Source: CAD feature listing. Evaluate the final solid. Frame: model axes, mm. Face numbers are marked on the shaded views. A direction names the side the tool comes from. Round coordinates to 2 decimals unless told otherwise and drop trailing zeros. Order: outer loops, then holes, each group sorted by start corner. A loop starts at its lowest first (then second) coordinate and runs counter-clockwise, first axis right, second up. Notation, with made-up numbers: M -19.75,-18.75 L 10.25,-18.75 A20 ccw 10.25,11.25 Z; hole C 47,15 d1. An arc over 180 degrees is marked long. Answer in a Markdown table with one row per item. Add a question column.
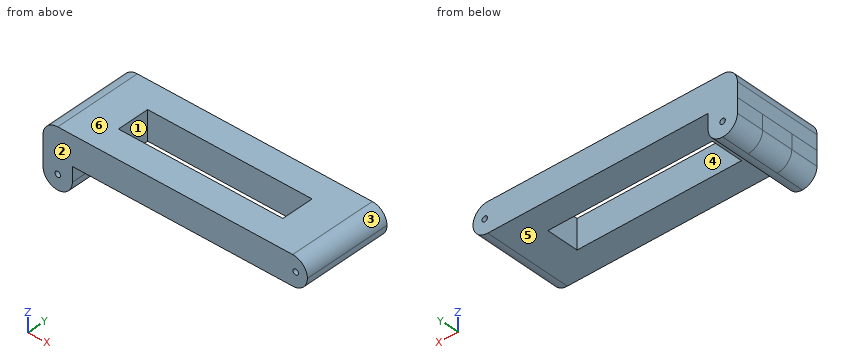
Autodesk Fusion 360 part; units mm, degrees
sketch "Esquisse1" plane through (0, 0, 0) normal (0, 0, 1) x (1, 0, 0)
  line L0 (-58.016, 25) -> (31.984, 25)
  line L1 (31.984, 25) -> (31.984, -5)
  line L2 (31.984, -5) -> (-58.016, -5)
  line L3 (-58.016, -5) -> (-58.016, 25)
  dimension "d1" = 90
  dimension "d2" = 30
extrude "Extrusion1" add sketch "Esquisse1" along normal blind 10
sketch "Esquisse11" plane through (0, 0, 0) normal (0, 1, 0) x (1, 0, 0)
  line L0 (-58.0163, -0.0111) -> (-48.0163, -0.0111)
  line L1 (-48.0163, -0.0111) -> (-48.0163, 9.9889)
  line L2 (-48.0163, 9.9889) -> (-58.0163, 9.9889)
  line L3 (-58.0163, 9.9889) -> (-58.0163, -0.0111)
  dimension "d56" = 10
  dimension "d57" = 10
extrude "Extrusion7" add sketch "Esquisse11" along normal blind 25 and the other way blind 5
sketch "Esquisse5" plane through (0, -5, 0) normal (0, -1, 0) x (1, 0, 0)
  line L0 (-48.0163, 0) -> (31.984, 0)
  line L1 (31.984, 0) -> (31.984, 10)
  line L2 (31.984, 10) -> (-58.016, 10)
  line L3 (-58.016, 10) -> (-58.016, 0.0111)
  circle A0 centre (28, 5) radius 6.5
  circle A1 centre (-53.0143, -5.2112) radius 7.25
  line L4 (-58.0163, 0.0111) -> (-58.0163, -9.9889)
  line L5 (-58.0163, -9.9889) -> (-48.0163, -9.9889)
  line L6 (-48.0163, -9.9889) -> (-48.0163, 0)
  line L7 (-58.016, 0.0111) -> (-58.0163, 0.0111)
  dimension "d11" = 13
  dimension "d46" = 14.5
sketch "Esquisse7" plane through (0, 0, 10) normal (0, 0, 1) x (-1, 0, 0)
  line L0 (-31.984, 5) -> (-31.984, -25)
  line L1 (-31.984, -25) -> (58.016, -25)
  line L2 (58.016, 5) -> (-31.984, 5)
  line L3 (41.016, -15.609) -> (-14.984, -15.609)
  line L4 (-14.984, -15.609) -> (-14.984, -4.609)
  line L5 (-14.984, -4.609) -> (41.016, -4.609)
  line L6 (41.016, -4.609) -> (41.016, -15.609)
  line L7 (58.016, -25) -> (58.016, 5)
  dimension "d47" = 11
  dimension "d48" = 56
  dimension "d49" = 17
extrude "Extrusion9" cut sketch "Esquisse5" along normal blind -9.5 and the other way blind 20.5 contours A1 L4 L5 L6 | L0 L1 L2 A0 picked at (-53.1071, -10.8113) picked at (32.8226, 5)
extrude "Extrusion4" cut sketch "Esquisse7" along normal blind 0 and the other way blind 10 contours L3 L4 L5 L6
sketch "Esquisse8" plane through (0, -5, 0) normal (0, -1, 0) x (1, 0, 0)
  line L0 (-48.0163, 0) -> (31.984, 0)
  line L1 (31.984, 0) -> (31.984, 10)
  line L2 (31.984, 10) -> (-58.016, 10)
  line L3 (-58.016, 10) -> (-58.016, 0.0111)
  circle A0 centre (-53, -5) radius 0.925
  line L4 (-58.016, 0.0111) -> (-58.0163, 0.0111)
  line L5 (-58.0163, 0.0111) -> (-58.0163, -9.9889)
  line L6 (-58.0163, -9.9889) -> (-48.0163, -9.9889)
  line L7 (-48.0163, -9.9889) -> (-48.0163, 0)
  dimension "d23" = 1.85
extrude "Extrusion5" cut sketch "Esquisse8" along normal blind 0 and the other way blind 30 contours A0
sketch "Esquisse9" plane through (0, -5, 0) normal (0, -1, 0) x (1, 0, 0)
  circle A0 centre (-53, -5) radius 0.925
  line L0 (-48.0163, 0) -> (31.984, 0)
  line L1 (31.984, 0) -> (31.984, 10)
  line L2 (31.984, 10) -> (-58.016, 10)
  line L3 (-58.016, 10) -> (-58.016, 0.0111)
  circle A1 centre (28, 5) radius 0.925
  line L4 (-58.016, 0.0111) -> (-58.0163, 0.0111)
  line L5 (-58.0163, 0.0111) -> (-58.0163, -9.9889)
  line L6 (-58.0163, -9.9889) -> (-48.0163, -9.9889)
  line L7 (-48.0163, -9.9889) -> (-48.0163, 0)
  dimension "d28" = 1.85
extrude "Extrusion6" cut sketch "Esquisse9" along normal blind 0 and the other way blind 30 contours A1
fillet "Congé8" radius 5 4 edges at (-58.0163, 20.25, -9.9889) (-58.0163, -0.25, -9.9889) (-48.0163, -0.25, -9.9889) (-48.0163, 20.25, -9.9889)
fillet "Congé9" radius 5 5 edges at (-58.016, 10, 10) (31.984, 20.25, 0) (31.984, -0.25, 0) (31.984, -0.25, 10) (31.984, 20.25, 10)
(1) Cut plane B-B (x = 28). Return loops of the section in (y, z) (3 decimals), and give its area (3 significant figures).
(2) Draft query along X for the marked faces 1, 2 and 3. Return one class per face: +X half, -X half, draft (parallel to the pull), parting line (faces both ways), or undercut.
(3) Access query for the marked faces 4, 5 and 6. Directions: +Z, -Z, +X, -X, +Y, -Y. A direction counts if a zero-diameter tool reaches every point of the face in a straight line with its end or side. Return the directions, or none.
(4) Pin query (flat end, axial travel): pin 1 (12 mm diameter, centred on x = -7.5, y = 20.5, fed in from -Z); pin 2 (5.5 mm diameter, centred on y = 17, z = -3, fed in from +X). Return the tip coordinate at first contact, or that it passes through.
(5) Line query: line 1 (X direction, y = 8.5, z = 4.75); line 2 (Y direction, x = -30.5, z = 5.25); line 3 (Z direction, x = 28, y = 14) (3 decimals). Output: solid intervals per line, ascending. Write a range as from..to.
(6) Cut plane D-D (z = -7.5). Return loops of the section in (x, y), and give its area (3 significant figures).
(7) Cut plane A-A (y = 8). Count the separate pieces of the cut face and the enclosed holes in it, and give its area (3 significant figures).
Answer list:
| question | item | result |
|---|---|---|
| 1 | outline | M -5,0.104 L 25,0.104 L 25,4.075 L -5,4.075 Z; M -5,5.925 L 25,5.925 L 25,9.896 L -5,9.896 Z |
| 1 | area | 238 mm² |
| 2 | face 1 | undercut |
| 2 | face 2 | draft |
| 2 | face 3 | +X half |
| 3 | face 4 | +Z, -Z |
| 3 | face 5 | -Z, +X, +Y, -Y |
| 3 | face 6 | +Z, +X, -X, +Y, -Y |
| 4 | pin 1 | z = 0 |
| 4 | pin 2 | x = -48.02 |
| 5 | line 1 | -58.02..-41.02, 14.98..27.11, 28.89..31.98 |
| 5 | line 2 | -5..4.61, 15.61..25 |
| 5 | line 3 | 0.104..4.075, 5.925..9.896 |
| 6 | outline | M -57.34,-5 L -48.69,-5 L -48.69,25 L -57.34,25 Z |
| 6 | area | 259 mm² |
| 7 | separate pieces | 2 |
| 7 | enclosed holes | 2 |
| 7 | area | 408 mm² |
